Here's how the part is built. I have some questions about the finished solid (model axes, mm). A direction names the side the tool comes from. Round coordinates to 2 decimals unless told otherwise and drop trailing zeros. Write each loop counter-clockwise with the first axis right and the second up, starting at its lowest first coordinate (ties: lowest second). Pieces come first, ordered by that corner, then holes. Notation, with made-up numbers: (-4.5, -36) - (39.5, -36) arc R24 cw to (39.5, -12) - close; hole circle Ø6 at (81.25, 56.5). An arc over 180 degrees is marked (long way). One line per item, written item: value. Start each with the question number.
Item 1: Imagine slicing it at A-A, the plane x = 50. Please give me the cut outline in (y, z).
Item 2: Imagine slicing it at C-C, the plane y = 16. Please give me the cut outline in (x, z), then the cut area to 4 significant figures.
Item 3: Imagine slicing it at B-B, the plane z = -116.5. Please give me the cut outline in (x, y).
Item 4: For P1, Ø1, axis at x = 65.5, y = 19, coming from the -Z side; P2, Ø4, axis at y = 29.5, z = -39, coming from the +X side; P3, Ø5, axis at x = 43, z = -55.5, coming from the +Y side; P4, Ø1.5, axis at y = 8, z = -74.5, coming from the +X side, each with a flat end and sliding along its axis, tell me the tip position at first contact or that it passes through.
Item 5: Imagine slicing it at D-D, the plane y = 36. Please give me the cut outline in (x, z).
Item 6: Thinking about a two-plate mould opening in X: for faces 4 (the face through (42, 0, -71)), 5 (the face through (42, 16, -3)), 6 (the face through (87.465, 4.737, -64.09)), 7 (the face through (-2.465, 4.737, -64.09)), which applies, released by +X, released by -X, zero draft, split by the parting line, or undercut?
Item 7: For faces 1 (the face through (0, 13, -66)), 2 (the face through (0, 32, -64)), 3 (the face through (41.84, 4.87, -4.74)), which set-ups out of +Z, -Z, +X, -X, +Y, -Y let a thin tool reach every point of the face, with its end or its side?
Item 8: If I drill on line 1 (X direction, y = 14, z = -88); line 2 (Y direction, x = 68.5, z = -72.5); line 3 (Z direction, x = 29, y = 22.5), over which ranges is the centre line in solid material (lowest first)?
```python
from build123d import *

# Parameters (mm, degrees)
SKETCH1_W                           = 85
SKETCH1_H                           = 130
BOSS_EXTRUDE1_BASE_DEPTH            = 3
BOSS_EXTRUDE4_SIDE_WALLS_DEPTH      = 130
CUT_EXTRUDE2_GUIDE_HOLES_DEPTH      = 163.616112363
SKETCH15_W                          = 85
SKETCH15_H                          = 20
BOSS_EXTRUDE9_FRONT_WALL_DEPTH      = 3
CHAMFER5_FRONT_CHAMFER_SIZE         = 9.61
CHAMFER6_FRONT_CHAMFER_CLEANUP_SIZE = 5
BOSS_EXTRUDE1_DEPTH                 = 130


with BuildPart() as part:
    # Sketch1 → Boss-Extrude1 _Base (new body)
    with BuildSketch(Plane(origin=(0, 0, 0), x_dir=(1, 0, 0), z_dir=(0, 1, 0))):
        with Locations((42.5, 65)):
            Rectangle(SKETCH1_W, SKETCH1_H)
    extrude(amount=BOSS_EXTRUDE1_BASE_DEPTH)

    # Sketch5 → Boss-Extrude4 _Side Walls (add, through all)
    with BuildSketch(Plane.XY):
        Polygon((-5, 28.390936655), (0, 38), (0, 0), (-5, 9.609063345), align=None)
        Polygon((90, 9.609063345), (90, 28.390936655), (85, 38), (85, 0), align=None)
    extrude(amount=-BOSS_EXTRUDE4_SIDE_WALLS_DEPTH)

    # Sketch4 → Cut-Extrude2 _Guide Holes (cut, through all)
    with BuildSketch(Plane.XY):
        Polygon((-3.1, 23), (0, 26.1), (0, 23), align=None)
        Polygon((85, 23), (88.1, 23), (85, 26.1), align=None)
    extrude(amount=-CUT_EXTRUDE2_GUIDE_HOLES_DEPTH, mode=Mode.SUBTRACT)

    # Sketch15 → Boss-Extrude9 _Front Wall (add)
    with BuildSketch(Plane.XY):
        with Locations((42.5, 13)):
            Rectangle(SKETCH15_W, SKETCH15_H)
    extrude(amount=-BOSS_EXTRUDE9_FRONT_WALL_DEPTH)

    # Chamfer5 _Front Chamfer
    chamfer5_front_chamfer_edges = [part.edges().sort_by_distance(p)[0] for p in [
        (42.5, 0, 0),
    ]]
    chamfer(chamfer5_front_chamfer_edges, length=CHAMFER5_FRONT_CHAMFER_SIZE)

    # Chamfer6 _Front Chamfer Cleanup
    chamfer6_front_chamfer_cleanup_edges = [part.edges().sort_by_distance(p)[0] for p in [
        (42.5, 3, -3),
    ]]
    chamfer(chamfer6_front_chamfer_cleanup_edges, length=CHAMFER6_FRONT_CHAMFER_CLEANUP_SIZE)

    # Sketch16 → Boss-Extrude1 (add, through all)
    with BuildSketch(Plane.XY):
        Polygon((0, 26.1), (0, 38.6), (-5, 28.390936655), align=None)
        Polygon((90, 28.390936655), (85, 26.1), (85, 38.6), align=None)
    extrude(amount=-BOSS_EXTRUDE1_DEPTH)


solid = part.part
```
Values follow:
1. outline: (0, -130) - (3, -130) - (3, -8) - (8, -3) - (23, -3) - (23, 0) - (9.61, 0) - (0, -9.61) - close
2. outline: (-5, -130) - (0, -130) - (0, -3) - (85, -3) - (85, -130) - (90, -130) - (90, 0) - (-5, 0) - close
2. area: 1,555 mm^2
3. outline: (-5, 9.61) - (0, 0) - (85, 0) - (90, 9.61) - (90, 28.39) - (85, 38.6) - (85, 26.1) - (88.1, 23) - (85, 23) - (85, 3) - (0, 3) - (0, 23) - (-3.1, 23) - (0, 26.1) - (0, 38.6) - (-5, 28.39) - close
4. P1: stops at z = -3
4. P2: stops at x = 90
4. P3: stops at y = 3
4. P4: stops at x = 89.55
5. outline: (-1.27, -130) - (0, -130) - (0, 0) - (-1.27, 0) - close; (85, -130) - (86.27, -130) - (86.27, 0) - (85, 0) - close
6. face 4: zero draft
6. face 5: undercut
6. face 6: released by +X
6. face 7: released by -X
7. face 1: -Z, +Y
7. face 2: +Z, -Z, +Y
7. face 3: +Z, +X, -X, -Y
8. line 1: x = -5 to 0, 85 to 90
8. line 2: y = 0 to 3
8. line 3: z = -3 to 0
